Read the model definition and answer for the solid it produces. Units are mm, in the model's axes. A direction names the side the tool comes from. Give positions to 0.01 mm unless a question says otherwise; leave off trailing zeros. Loops run counter-clockwise (first coordinate to the right, second up) from the corner with the lowest first, then second, coordinate; pieces in that order, holes last. Notation, with made-up numbers: (81, 76) - (139, 76) arc R4 ccw to (139, 82) - close; hole circle Ø8 at (-0.5, 83.25). An arc over 180 degrees is marked (long way). Write item = value, one per line.
```python
from build123d import *

# Parameters (mm, degrees)
SCHIZZO1_W                   = 60
SCHIZZO1_H                   = 60
ESTRUSIONE_ESTRUSIONE1_DEPTH = 10


with BuildPart() as part:
    # Schizzo1 → Estrusione-Estrusione1 (new body)
    with BuildSketch(Plane.XY):
        Rectangle(SCHIZZO1_W, SCHIZZO1_H)
        Polygon((0, -25), (25, 0), (0, 25), (-25, 0), align=None, mode=Mode.SUBTRACT)
    extrude(amount=ESTRUSIONE_ESTRUSIONE1_DEPTH)


solid = part.part
```
1) A cutting plane is placed at B-B on y = 11.5. Determine the outline of the cut face in (x, z), then the cut area to 3 significant figures.
Output:
outline = (-30, 0) - (-13.5, 0) - (-13.5, 10) - (-30, 10) - close; (13.5, 0) - (30, 0) - (30, 10) - (13.5, 10) - close
area = 330 mm²
2) A cutting plane is placed at A-A on x = 7.5. Determine the outline of the cut face in (y, z), then the cut area to 3 significant figures.
Output:
outline = (-30, 0) - (-17.5, 0) - (-17.5, 10) - (-30, 10) - close; (17.5, 0) - (30, 0) - (30, 10) - (17.5, 10) - close
area = 250 mm²
3) A cutting plane is placed at C-C on z = 6. Determine the outline of the cut face in (x, y), then the cut area to 3 significant figures.
Output:
outline = (-30, -30) - (30, -30) - (30, 30) - (-30, 30) - close; hole (-25, 0) - (0, -25) - (25, 0) - (0, 25) - close
area = 2,350 mm²
4) Find the intervals of material crossed by probe 1 along X at (y, z) = (5, 3.75); probe 2 along X at (y, z) = (9, 8.5); probe 3 along Y at (x, z) = (11, 2.5), in increasing order.
Output:
probe_1 = -30 to -20, 20 to 30
probe_2 = -30 to -16, 16 to 30
probe_3 = -30 to -14, 14 to 30
5) A tool of negligible diameter and unlimited length cuts with its end or side. For faces 1 (the face through (12, -13, 5)), 2 (the face through (-14, 14, 0)), from which of +Z, -Z, +X, -X, +Y, -Y can it reach the whole face along a straight path? Write none if from no direction.
Output:
face_1 = +Z, -Z
face_2 = -Z, +X, -X, +Y, -Y
